Read the model definition and answer for the solid it produces. Units are mm, in the model's axes. A direction names the side the tool comes from. Give positions to 0.01 mm unless a question says otherwise; leave off trailing zeros. Loops run counter-clockwise (first coordinate to the right, second up) from the corner with the lowest first, then second, coordinate; pieces in that order, holes last. Notation, with made-up numbers: (1.5, -2) -> (35.5, -2) arc R5 ccw to (35.5, 6) -> close; hole circle Ø8 at (-25, -15). An arc over 180 degrees is marked (long way). One line per item, written item: value. Start each with the question number.
from build123d import *

# Parameters (mm, degrees)
BOSS_EXTRUDE1_START = -10
SKETCH1_W           = 12
SKETCH1_H           = 10
BOSS_EXTRUDE1_DEPTH = 20
BOSS_EXTRUDE2_START = -3.6
SKETCH2_W           = 7.2
SKETCH2_H           = 5
BOSS_EXTRUDE2_DEPTH = 7.2
BOSS_EXTRUDE3_START = -7.8
SKETCH3_W           = 1.6
SKETCH3_H           = 12
BOSS_EXTRUDE3_DEPTH = 1.6
BOSS_EXTRUDE4_START = 6.2
SKETCH4_W           = 1.6
SKETCH4_H           = 12
BOSS_EXTRUDE4_DEPTH = 1.6
BOSS_EXTRUDE5_START = -55
SKETCH5_R           = 3.5
BOSS_EXTRUDE5_DEPTH = 46


with BuildPart() as part:
    # Sketch1 → Boss-Extrude1 (new body)
    with BuildSketch(Plane.XY.offset(BOSS_EXTRUDE1_START)):
        with Locations((0, 5)):
            Rectangle(SKETCH1_W, SKETCH1_H)
    extrude(amount=BOSS_EXTRUDE1_DEPTH)


with BuildPart() as body_2:
    # Sketch2 → Boss-Extrude2 (new body)
    with BuildSketch(Plane.XY.offset(BOSS_EXTRUDE2_START)):
        with Locations((0, 1.5)):
            Rectangle(SKETCH2_W, SKETCH2_H)
    extrude(amount=BOSS_EXTRUDE2_DEPTH)


with BuildPart() as part_1:
    add(part.part)

    # Combine1: cut body 2
    add(body_2.part, mode=Mode.SUBTRACT)


with BuildPart() as body_2_2:
    # Sketch3 → Boss-Extrude3 (new body)
    with BuildSketch(Plane.XY.offset(BOSS_EXTRUDE3_START)):
        with Locations((0, 5)):
            Rectangle(SKETCH3_W, SKETCH3_H)
    extrude(amount=BOSS_EXTRUDE3_DEPTH)


with BuildPart() as part_2:
    add(part_1.part)

    # Combine2: cut body 2 2
    add(body_2_2.part, mode=Mode.SUBTRACT)


with BuildPart() as body_2_3:
    # Sketch4 → Boss-Extrude4 (new body)
    with BuildSketch(Plane.XY.offset(BOSS_EXTRUDE4_START)):
        with Locations((0, 5)):
            Rectangle(SKETCH4_W, SKETCH4_H)
    extrude(amount=BOSS_EXTRUDE4_DEPTH)


with BuildPart() as part_3:
    add(part_2.part)

    # Combine3: cut body 2 3
    add(body_2_3.part, mode=Mode.SUBTRACT)

    # Sketch5 → Boss-Extrude5 (add)
    with BuildSketch(Plane.XY.offset(BOSS_EXTRUDE5_START)):
        with Locations(Location((0, 6, 0), (0, 0, 180))):
            Circle(SKETCH5_R)
    extrude(amount=BOSS_EXTRUDE5_DEPTH)


solid = part_3.part
Item 1: Section B-B, the plane x = 0 is taken. Determine the outline of the cut face in (y, z), plus the area to 3 significant figures.
Item 2: For faces 1 (the flat face through (0, 5, -6.2)), 2 (the flat face through (0, 2, -3.6)), 3 (the flat face through (0, 2, -10)), determine the directions among +Z, -Z, +X, -X, +Y, -Y from which every point of the face is accessible in a straight line to the end or side of a thin tool.
Item 3: Flat-ended cylindrical pins translate along their axes: pin 1 (1.2 mm diameter, centred on x = -1, y = 1, fed in from -Z); pin 2 (6 mm diameter, centred on x = -3, z = 1, fed in from -Y); pin 3 (1 mm diameter, centred on y = 9, z = -19, fed in from +X); pin 4 (1.5 mm diameter, centred on y = 3.5, z = -30.5, fed in from -X). Find the tip coordinate at first contact, or state that the pin passes through.
Item 4: Section A-A, the plane y = 6 is taken. Determine the outline of the cut face in (x, z).
Item 5: Determine the mould class of faces 4 (the flat face through (3.6, 2, 0)), 5 (the flat face through (6, 5, 0)), 6 (the flat face through (-6, 5, 0)) for opening direction X: pulls with the +X half, pulls with the -X half, needs draft (parallel to the pull), parting line crosses it, or undercut.
Item 6: Consider L1, parallel to Z at x = 0.25, y = 3; L2, parallel to Z at x = 0.75, y = 8; L3, parallel to Z at x = 1.25, y = 1. Determine where each line is inside the solid, lowest interval first. Write a range as [from, to].
Item 7: Section D-D, the plane x = 2.75 is taken. Determine the outline of the cut face in (y, z).
Item 8: Section C-C, the plane z = -48.5 is taken. Determine the outline of the cut face in (x, y), plus the area to 3 significant figures.
Computed values:
1. outline: (0, -10) -> (2.5, -10) -> (2.5, -55) -> (9.5, -55) -> (9.5, -10) -> (10, -10) -> (10, -7.8) -> (0, -7.8) -> close; (0, -6.2) -> (10, -6.2) -> (10, 6.2) -> (0, 6.2) -> (0, 3.6) -> (4, 3.6) -> (4, -3.6) -> (0, -3.6) -> close; (0, 7.8) -> (10, 7.8) -> (10, 10) -> (0, 10) -> close
1. area: 454 mm²
2. face 1: +Y, -Y
2. face 2: -Y
2. face 3: -Z
3. pin 1: z = -10
3. pin 2: y = 0
3. pin 3: x = 2.45
3. pin 4: x = -3.03
4. outline: (-6, -10) -> (-3.5, -10) -> (-3.5, -55) -> (3.5, -55) -> (3.5, -10) -> (6, -10) -> (6, 10) -> (-6, 10) -> close; hole (-0.8, -7.8) -> (0.8, -7.8) -> (0.8, -6.2) -> (-0.8, -6.2) -> close; hole (-0.8, 6.2) -> (0.8, 6.2) -> (0.8, 7.8) -> (-0.8, 7.8) -> close
5. face 4: undercut
5. face 5: pulls with the +X half
5. face 6: pulls with the -X half
6. L1: [-55, -7.8], [-6.2, -3.6], [3.6, 6.2], [7.8, 10]
6. L2: [-55, -7.8], [-6.2, 6.2], [7.8, 10]
6. L3: [-10, -3.6], [3.6, 10]
7. outline: (0, -10) -> (3.83, -10) -> (3.83, -55) -> (8.17, -55) -> (8.17, -10) -> (10, -10) -> (10, 10) -> (0, 10) -> (0, 3.6) -> (4, 3.6) -> (4, -3.6) -> (0, -3.6) -> close
8. outline: circle Ø7 at (0, 6)
8. area: 38.5 mm²
